Geometry check sheet. Reference: the model listing, model coordinates, mm. A direction names the side the tool comes from. Coordinates: 2 decimals unless noted, no trailing zeros. Loops run counter-clockwise (first coordinate to the right, second up) from the corner with the lowest first, then second, coordinate; pieces in that order, holes last. Notation, with made-up numbers: (-34.5, 74) -> (22.5, 74) arc R13 ccw to (22.5, 79) -> close; hole circle Ø9 at (-26.5, 29.5). An arc over 180 degrees is marked (long way). Answer as a JSON object with one key per item and string values.
from build123d import *

# Parameters (mm, degrees)
F1_DEPTH  = 63.5
F2_DEPTH  = 50.8
F3_DEPTH  = 7.9375
F2_FACE_W = 50.8
F2_FACE_H = 18.2610141082


with BuildPart() as f1:
    # F0 (on Front) → F1 (new body, symmetric)
    with BuildSketch(Plane.XZ):
        Polygon((22.225, 9.525), (-41.275, 9.525), (-41.275, -9.525), (41.275, -9.525), (41.275, 9.525), align=None)
    extrude(amount=F1_DEPTH, both=True)

    # F0 (on Front) → F2 (join)
    with BuildSketch(Plane.XZ):
        with BuildLine():
            Line((22.225, 33.7634080377), (22.225, 9.525))
            Line((22.225, 9.525), (41.275, 9.525))
            Line((41.275, 9.525), (41.275, 33.7634080377))
            ThreePointArc((41.275, 33.7634080377), (45.8279770824, 44.8911850867), (56.8753051405, 49.636031253))
            Line((56.8753051405, 49.636031253), (56.8753051405, 67.8970453611))
            add(Edge.make_bspline(
                [(57.15, 68.6884080377), (57.335632748, 68.5042193152), (57.0807165436, 68.2374790668), (56.8753051405, 67.8970453611)],
                knots=[0.9213128399, 0.9213128399, 0.9213128399, 0.9213128399, 1, 1, 1, 1], degree=3))
            ThreePointArc((57.15, 68.6884080377), (32.4542956671, 58.4591123706), (22.225, 33.7634080377))
        make_face()
    extrude(amount=F2_DEPTH)

    # F0 (on Front) → F3 (join, symmetric)
    with BuildSketch(Plane.XZ):
        with BuildLine():
            add(Edge.make_bspline(
                [(-41.275, 9.525), (-7.5919390656, 61.6845674813), (54.9765090021, 70.8449915853), (57.15, 68.6884080377)],
                knots=[0, 0, 0, 0, 0.9213128399, 0.9213128399, 0.9213128399, 0.9213128399], degree=3))
            Line((-41.275, 9.525), (22.225, 9.525))
            Line((22.225, 9.525), (22.225, 33.7634080377))
            ThreePointArc((22.225, 33.7634080377), (32.4542956671, 58.4591123706), (57.15, 68.6884080377))
        make_face()
    extrude(amount=F3_DEPTH, both=True)

    # F2_face (on face) → F4 (revolve)
    with BuildSketch(Plane(origin=(56.8753051405, -25.4, 58.7665383071), x_dir=(0, 1, 0), z_dir=(1, 0, 0))):
        Rectangle(F2_FACE_W, F2_FACE_H)
    revolve(axis=Axis((56.8753051405, 0, 58.7665383071), (0, 0, -1)))


solid = f1.part
1. Thickness scan on probe 1 along X at (y, z) = (57.5, 6) (3 decimals); probe 2 along Z at (x, y) = (-29.5, 35) (3 decimals); probe 3 along Z at (x, y) = (62, 3). Record the ranges inside material, lowest first. Write a range as from..to.
Evaluation:
{"probe 1": "x = -41.275..41.275", "probe 2": "z = -9.525..9.525", "probe 3": "z = 49.64..67.9"}
2. Section check C-C, the plane x = 98. Record the boundary of the cut face in (y, z), then the cut area to 3 significant figures.
Evaluation:
{"outline": "(-29.82, 49.64) -> (29.82, 49.64) -> (29.82, 67.9) -> (-29.82, 67.9) -> close", "area": "1,090 mm^2"}
3. Depth check by flat-ended pin: P1, Ø5, axis at x = 83.5, y = -18, coming from the +Z side; P2, Ø4, axis at y = 3.5, z = 16, coming from the +X side (3 decimals); P3, Ø17.5, axis at x = 48, z = 29, coming from the +Y side. Enter the tip coordinate at first touch or a pass-through.
Evaluation:
{"P1": "stops at z = 67.9", "P2": "stops at x = 22.225", "P3": "stops at y = 0"}
4. Section check B-B, the plane z = 57.5. Record the boundary of the cut face in (x, y), then the cut area to 3 significant figures.
Evaluation:
{"outline": "(31.53, -50.8) -> (56.88, -50.8) arc R50.8 ccw (long way) to (31.53, -44.03) -> close", "area": "8,160 mm^2"}
5. Section check A-A, the plane y = -55.5. Record the boundary of the cut face in (x, z) (3 decimals).
Evaluation:
{"outline": "(-41.275, -9.525) -> (41.275, -9.525) -> (41.275, 9.525) -> (-41.275, 9.525) -> close"}
6. Tool access check on faces 4 (the face through (36, -50.8, 40)), 5 (the face through (58.26, 50.78, 58.89)), 6 (the face through (23.165, 3.913, 41.814)), 7 (the face through (41.275, -15, 7)). Record the directions out of +Z, -Z, +X, -X, +Y, -Y that give a thin tool (end or side, any length) a straight path to the whole face; none if there is none.
Evaluation:
{"face 4": "+Z, +X, -X, -Y", "face 5": "+Z", "face 6": "+X, +Y", "face 7": "-Z, +X, +Y, -Y"}
7. Mould release check, pull along Z, two halves, no side actions. Record for faces 1 (the face through (-1, -1, -9.525)), 2 (the face through (-41.275, -1, 0)), 3 (the face through (0, 7.938, 27)): released by +Z, released by -Z, zero draft, split by the parting line, or undercut.
Evaluation:
{"face 1": "released by -Z", "face 2": "zero draft", "face 3": "undercut"}
